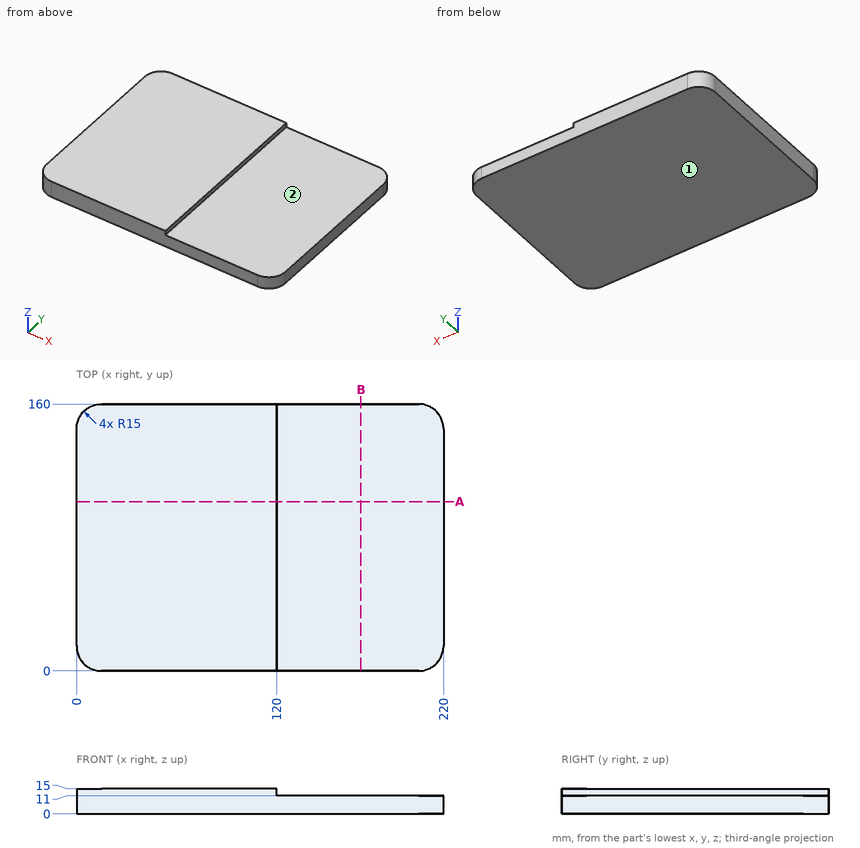
The figure shows three views and two pictorial views of one solid part (mm, origin at its lowest corner). Answer the questions. A direction names the side the tool comes from. Coordinates: 2 decimals unless noted, no trailing zeros. Loops run counter-clockwise (first coordinate to the right, second up) from the corner with the lowest first, then second, coordinate; pieces in that order, holes last. Notation, with made-up numbers: (30.5, 73) -> (42.5, 73) arc R23 cw to (42.5, 94) -> close; hole circle Ø6 at (-20, 75). An arc over 180 degrees is marked (long way). Write item = value, one per line. Start each with the question number.
1) A tool of negligible diameter and unlimited length cuts with its end or side. For the marked faces 1 and 2, from which of +Z, -Z, +X, -X, +Y, -Y can it reach the whole face along a straight path? Write none if from no direction.
2) A cutting plane is placed at A-A (y = 101.5). Give the vertices of the cut face in (x, z), then the cut area to 3 significant figures.
3) A cutting plane is placed at B-B (x = 170.5). Give the vertices of the cut face in (y, z).
4) Straight lines are drawn through the part: line 1 (Z direction, x = 140.5, y = 83); line 2 (Y direction, x = 206, z = 7.5); line 3 (X direction, y = 65, z = 14). For each, find the intervals that lie inside material, in ascending order. Write a range as from..to.
5) Given pin 1 Ø1.5 at (x, y) = (117, 65.5) entering from -Z, flat-ended and moving along its own axis, determine where the tip first touches the part or whether it passes through.
Responses:
q1.face_1 = -Z, +X, -X, +Y, -Y
q1.face_2 = +Z, +X, +Y, -Y
q2.outline = (0, 0) -> (220, 0) -> (220, 11) -> (120, 11) -> (120, 15) -> (0, 15) -> close
q2.area = 2,900 mm²
q3.outline = (0, 0) -> (160, 0) -> (160, 11) -> (0, 11) -> close
q4.line_1 = 0..11
q4.line_2 = 0.03..159.97
q4.line_3 = 0..120
q5.pin_1 = 0
